Can you work these out from the drawing? Everything is in mm from the part's minimum corner. A direction names the side the tool comes from. Coordinates: 2 decimals unless noted, no trailing zeros. Loops run counter-clockwise (first coordinate to the right, second up) from the corner with the lowest first, then second, coordinate; pieces in that order, holes last.
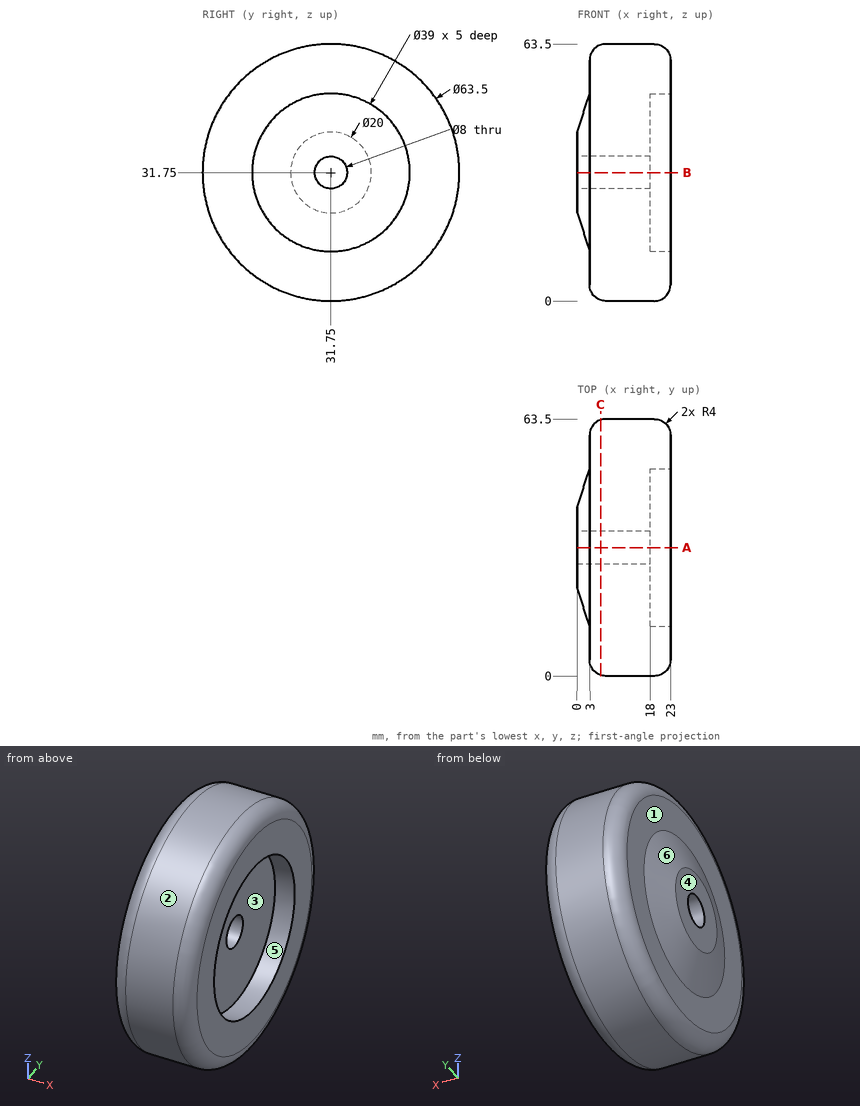
1. We'd pull the mould along Y, two halves only. Please class the marked faces 3, 4, 5 and 6: +Y half, -Y half, draft (parallel to the pull), parting line (faces both ways), or undercut.
2. I want a section at C-C (x = 5.75). Please give me the cut outline in (y, z), then the cut area to 3 significant figures.
3. I want a section at A-A (y = 31.75). Please give me the cut outline in (x, z).
4. I need wall thicknesses on line 1 along Z through (x, y) = (20, 23); line 2 along X through (y, z) = (41, 53.5); line 3 along Y through (x, z) = (20, 36.5). Which ranges of each line are inside material? Lowest first, please.
5. For pin 1 (6 mm diameter, centred on y = 9, z = 40.5, fed in from -X); pin 2 (1 mm diameter, centred on x = 14, y = 15, fed in from +Z); pin 3 (4 mm diameter, centred on x = 5.5, z = 23.5, fed in from -Y); pin 4 (6.5 mm diameter, centred on y = 31.75, z = 31.75, fed in from +X), each with a flat end and sliding along its axis, tell me the tip position at first contact or that it passes through.
6. On a 3-axis mill with a long thin cutter (end or side, diameter ignored), from which of +Z, -Z, +X, -X, +Y, -Y can I reach the whole of each face in a straight line? I mean the marked faces 1 and 2. Say none if no direction works.
Response values:
1. face 3: undercut
1. face 4: draft
1. face 5: undercut
1. face 6: parting line
2. outline: circle Ø63.1 at (31.75, 31.75); hole circle Ø8 at (31.75, 31.75)
2. area: 3,080 mm2
3. outline: (0, 21.75) - (3, 12.25) - (3, 4) arc R4 ccw to (7, 0) - (19, 0) arc R4 ccw to (23, 4) - (23, 12.25) - (18, 12.25) - (18, 27.75) - (0, 27.75) - close; (0, 35.75) - (18, 35.75) - (18, 51.25) - (23, 51.25) - (23, 59.5) arc R4 ccw to (19, 63.5) - (7, 63.5) arc R4 ccw to (3, 59.5) - (3, 51.25) - (0, 41.75) - close
4. line 1: z = 1.36 to 14.32, 49.18 to 62.14
4. line 2: x = 3 to 23
4. line 3: y = 0.49 to 12.84, 50.66 to 63.01
5. pin 1: stops at x = 3
5. pin 2: stops at z = 59.03
5. pin 3: stops at y = 0.71
5. pin 4: passes through
6. face 1: -X
6. face 2: +X, -X
